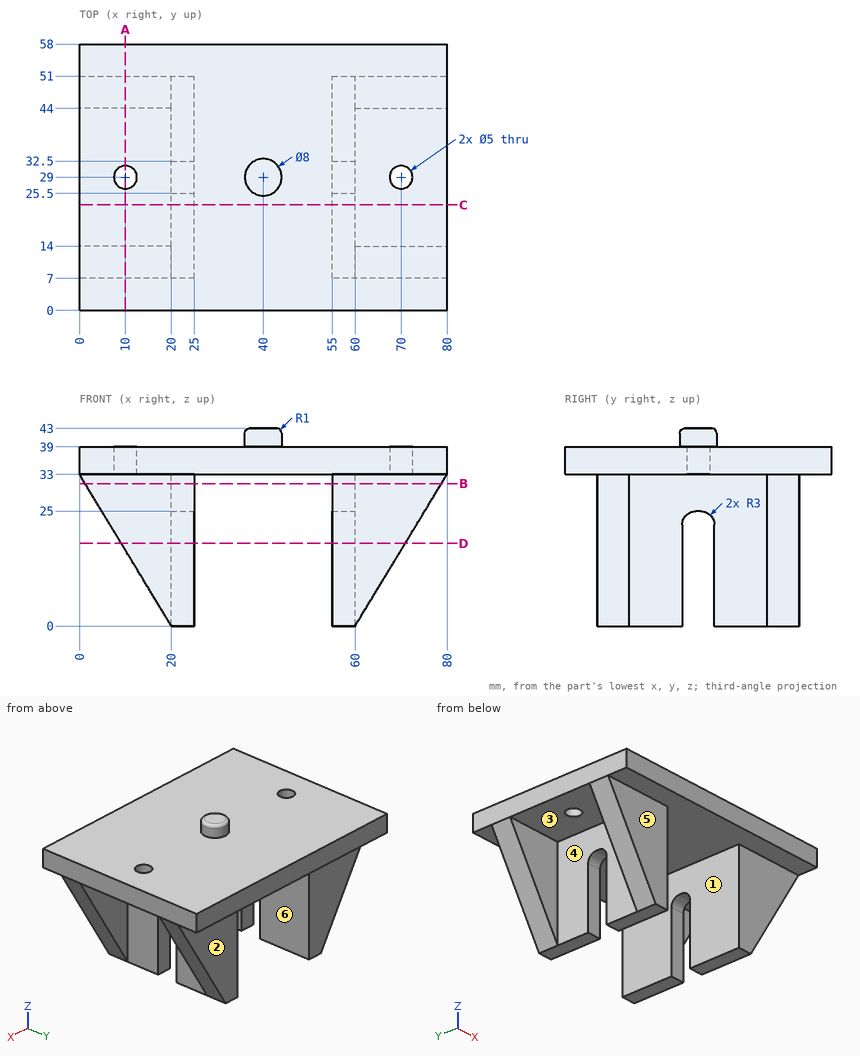
Check sheet for the drawn part. Datum: minimum x, y, z corner. Units: mm. A direction names the side the tool comes from. Round coordinates to 2 decimals unless told otherwise and drop trailing zeros. Order: outer loops, then holes, each group sorted by start corner. A loop starts at its lowest first (then second) coordinate and runs counter-clockwise, first axis right, second up. Notation, with made-up numbers: M -8,72.5 L 25,72.5 A12 ccw 25,84.5 Z; hole C 13.25,-18.5 d4. An arc over 180 degrees is marked long. Answer in a Markdown table with one row per item.
(1) Section check A-A on x = 10. Record the boundary of the cut face in (y, z).
Findings:
| item | result |
|---|---|
| outline | M 0,33 L 7,33 L 7,16.5 L 14,16.5 L 14,33 L 26.5,33 L 26.5,39 L 0,39 Z; M 31.5,33 L 44,33 L 44,16.5 L 51,16.5 L 51,33 L 58,33 L 58,39 L 31.5,39 Z |
(2) Gauge pin test, flat ends, axial feed: pin 1 (5.5 mm diameter, centred on x = 23.5, z = 9.5, fed in from +Y); pin 2 (5.5 mm diameter, centred on x = 57.5, z = 15, fed in from -Y); pin 3 (8 mm diameter, centred on x = 59.5, y = 22.5, fed in from +Z). Record the tip position at first contact, or that the pin passes through.
Findings:
| item | result |
|---|---|
| pin 1 | stops at y = 51 |
| pin 2 | stops at y = 7 |
| pin 3 | stops at z = 39 |
(3) Section check C-C on y = 23. Record the boundary of the cut face in (x, z).
Findings:
| item | result |
|---|---|
| outline | M 0,33 L 20,33 L 20,0 L 25,0 L 25,33 L 55,33 L 55,0 L 60,0 L 60,33 L 80,33 L 80,39 L 0,39 Z |
(4) Section check D-D on z = 18. Record the boundary of the cut face in (x, y).
Findings:
| item | result |
|---|---|
| outline | M 9.09,7 L 25,7 L 25,25.5 L 20,25.5 L 20,14 L 9.09,14 Z; M 9.09,44 L 20,44 L 20,32.5 L 25,32.5 L 25,51 L 9.09,51 Z; M 55,7 L 70.91,7 L 70.91,14 L 60,14 L 60,25.5 L 55,25.5 Z; M 55,32.5 L 60,32.5 L 60,44 L 70.91,44 L 70.91,51 L 55,51 Z |
(5) Material ranges on line 1 along Y through (x, z) = (70, 35.45); line 2 along Y through (x, z) = (65, 10); line 3 along X through (y, z) = (34, 22), recorded low to high. Write a range as from..to.
Findings:
| item | result |
|---|---|
| line 1 | y = 0..26.5, 31.5..58 |
| line 2 | y = 7..14, 44..51 |
| line 3 | x = 20..25, 55..60 |
(6) Section check B-B on z = 31. Record the boundary of the cut face in (x, y), plus the area to 3 significant figures.
Findings:
| item | result |
|---|---|
| outline | M 1.21,7 L 25,7 L 25,51 L 1.21,51 L 1.21,44 L 20,44 L 20,14 L 1.21,14 Z; M 55,7 L 78.79,7 L 78.79,14 L 60,14 L 60,44 L 78.79,44 L 78.79,51 L 55,51 Z |
| area | 966 mm^2 |
(7) Set-up check for the marked faces 1, 2 and 3: record each of +Z, -Z, +X, -X, +Y, -Y from which the full face is reachable in a straight line by a thin tool's end or side.
Findings:
| item | result |
|---|---|
| face 1 | -Z, +Y, -Y |
| face 2 | -Z, +X, -X, +Y |
| face 3 | -Z, -X |
(8) Draft check along Y on the marked faces 4, 5 and 6. Enter one of: +Y half, -Y half, draft (parallel to the pull), parting line (faces both ways), or undercut.
Findings:
| item | result |
|---|---|
| face 4 | undercut |
| face 5 | -Y half |
| face 6 | draft |
